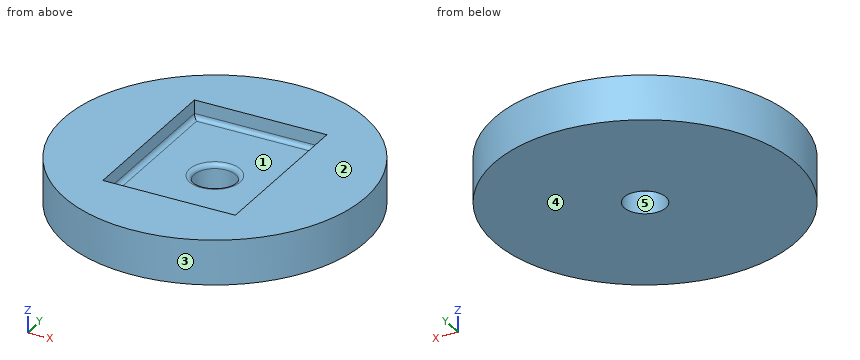
```python
from build123d import *

# Parameters (mm, degrees)
F0_R     = 42.7770323115
F1_DEPTH = 12.7
F2_W     = 37.5254675746
F2_H     = 47.488167882
F3_DEPTH = 5.08
F4_R     = 5.9019782965
F5_DEPTH = 25.4
F6_R     = 1.27


with BuildPart() as f1:
    # F0 (on Top) → F1 (new body)
    with BuildSketch(Plane.XY):
        Circle(F0_R)
    extrude(amount=F1_DEPTH)

    # F2 (on face) → F3 (cut)
    with BuildSketch(Plane.XY.offset(12.7)):
        Rectangle(F2_W, F2_H)
    extrude(amount=-F3_DEPTH, mode=Mode.SUBTRACT)

    # F4 (on face) → F5 (cut)
    with BuildSketch(Plane.XY.offset(7.62)):
        Circle(F4_R)
    extrude(amount=-F5_DEPTH, mode=Mode.SUBTRACT)

    # F6
    f6_edges = [f1.edges().sort_by_distance(p)[0] for p in [
        (0, 23.744084, 7.62),
        (18.762734, 0, 7.62),
        (0, -23.744084, 7.62),
        (-18.762734, 0, 7.62),
        (-5.901978, 0, 7.62),
    ]]
    fillet(f6_edges, radius=F6_R)


solid = f1.part
```
Geometry: final body of the model. Coordinates: model frame, mm. Face numbers are marked on the shaded views. A direction names the side the tool comes from. Round coordinates to 2 decimals unless told otherwise and drop trailing zeros. Write each loop counter-clockwise with the first axis right and the second up, starting at its lowest first coordinate (ties: lowest second). Pieces come first, ordered by that corner, then holes. Notation, with made-up numbers: M -6,-6.75 L 6,-6.75 A18 cw 6,16.25 Z; hole C 5,-20.5 d3. An arc over 180 degrees is marked long. Answer in a Markdown table with one row per item. Add a question column.
(1) Cut plane C-C, the plane z = 11.5. Return the cut outline in (x, y), then the cut area to 3 significant figures.
(2) Cut plane A-A, the plane x = 0. Return the cut outline in (y, z), then the cut area to 3 significant figures.
(3) Reachability of the marked faces 1 and 2 from +Z, -Z, +X, -X, +Y, -Y: full face, straight path, thin tool, end or side. Return the list, or none.
(4) Contact query for flat-ended pins moving along their axis: pin 1 (3 mm diameter, centred on y = -3.5, z = 10, fed in from -X); pin 2 (1.9 mm diameter, centred on x = 0, z = 11.5, fed in from -Y); pin 3 (5 mm diameter, centred on y = -23, z = 9, fed in from -X). Output: stop coordinate, or through.
(5) Cut plane B-B, the plane y = 0. Return the cut outline in (x, z), then the cut area to 3 significant figures.
(6) Cut plane D-D, the plane y = -34. Return the cut outline in (x, z).
(7) Draft query along Y for the marked faces 3, 4 and 5. Return one class per face: pulls with the +Y half, pulls with the -Y half, needs draft (parallel to the pull), parting line crosses it, or undercut.
(8) Ray query, L1, parallel to Y at x = 0, z = 1.5; L2, parallel to Y at x = 0.5, z = 11.75; L3, parallel to X at y = -4.5, z = 10.5. Return the intervals inside material, ascending.
Established:
| question | item | result |
|---|---|---|
| 1 | outline | C 0,0 d85.55; hole M -18.76,-23.74 L 18.76,-23.74 L 18.76,23.74 L -18.76,23.74 Z |
| 1 | area | 3,970 mm² |
| 2 | outline | M -42.78,0 L -5.9,0 L -5.9,6.35 A1.27 ccw -7.17,7.62 L -22.47,7.62 A1.27 cw -23.74,8.89 L -23.74,12.7 L -42.78,12.7 Z; M 5.9,0 L 42.78,0 L 42.78,12.7 L 23.74,12.7 L 23.74,8.89 A1.27 cw 22.47,7.62 L 7.17,7.62 A1.27 ccw 5.9,6.35 Z |
| 2 | area | 755 mm² |
| 3 | face 1 | +Z |
| 3 | face 2 | +Z, +X, -X, +Y, -Y |
| 4 | pin 1 | x = -42.73 |
| 4 | pin 2 | y = -42.78 |
| 4 | pin 3 | x = -37.54 |
| 5 | outline | M -42.78,0 L -5.9,0 L -5.9,6.35 A1.27 ccw -7.17,7.62 L -17.49,7.62 A1.27 cw -18.76,8.89 L -18.76,12.7 L -42.78,12.7 Z; M 5.9,0 L 42.78,0 L 42.78,12.7 L 18.76,12.7 L 18.76,8.89 A1.27 cw 17.49,7.62 L 7.17,7.62 A1.27 ccw 5.9,6.35 Z |
| 5 | area | 806 mm² |
| 6 | outline | M -25.96,0 L 25.96,0 L 25.96,12.7 L -25.96,12.7 Z |
| 7 | face 3 | parting line crosses it |
| 7 | face 4 | needs draft |
| 7 | face 5 | undercut |
| 8 | L1 | -42.78 to -5.9, 5.9 to 42.78 |
| 8 | L2 | -42.77 to -23.74, 23.74 to 42.77 |
| 8 | L3 | -42.54 to -18.76, 18.76 to 42.54 |
